from build123d import *

# Parameters (mm, degrees)
F3_W           = 1.8520833333
F3_H           = 3.7041666667
F3_H_2         = 3.175
F4_DEPTH       = 38.1
F6_DEPTH       = 25.401
F7_R           = 3.175
F8_DEPTH       = 15.24
F9_R           = 1.27
F10_DEPTH      = 22.225
F11_W          = 3.175
F11_H          = 3.81
F11_H_2        = 6.985
F12_DEPTH      = 3.175
F13_DEPTH      = 4.7625
F13_DEPTH_BACK = 3.175
F15_DEPTH      = 3.175


# Not quite as in the source:
# - a length typed as a fraction of an inch, garbled in the dataset ("3 / 203.2 mm" for 3/8 in), is restored
# - a feature names something its author has since deleted; it is built from what else it names


with BuildPart() as f1:
    # F0 (on Front) → F1 (revolve)
    with BuildSketch(Plane.XZ):
        Polygon((-38.1, 0), (-31.75, 0), (-31.75, 3.175), (-34.925, 3.175), (-34.925, 25.4), (-38.1, 25.4), align=None)
    revolve(axis=Axis((0, 0, 12.7), (0, 0, 1)))

    # F3 (on offset) → F4 (cut, symmetric)
    with BuildSketch(Plane.XZ.offset(38.1)):
        with Locations((-0.9260416667, 5.0270833333)):
            Rectangle(F3_W, F3_H)
        with Locations((0.9260416667, 5.0270833333)):
            Rectangle(F3_W, F3_H)
        with Locations((0.9260416667, 12.4354166667)):
            Rectangle(F3_W, F3_H)
        with Locations((-0.9260416667, 12.4354166667)):
            Rectangle(F3_W, F3_H)
        with Locations((-0.9260416667, 19.84375)):
            Rectangle(F3_W, F3_H)
        Polygon((1.8520833333, 3.175), (1.8520833333, 0), (50.8, 0), (50.8, 25.4), (1.8520833333, 25.4), (1.8520833333, 21.6958333333), (1.8520833333, 17.9916666667), (1.8520833333, 14.2875), (1.8520833333, 10.5833333333), (1.8520833333, 6.8791666667), align=None)
        with Locations((0.9260416667, 19.84375)):
            Rectangle(F3_W, F3_H)
        with Locations((0.9260416667, 1.5875)):
            Rectangle(F3_W, F3_H_2)
        with Locations((-0.9260416667, 1.5875)):
            Rectangle(F3_W, F3_H_2)
    extrude(amount=F4_DEPTH, both=True, mode=Mode.SUBTRACT)

    # F5 (on face) → F6 (cut, through all)
    with BuildSketch(Plane.XY.offset(25.4)):
        with BuildLine():
            ThreePointArc((0, 38.1), (3.175, 34.925), (0, 31.75))
            ThreePointArc((0, 31.75), (22.4506403027, 22.4506403027), (31.75, 0))
            Line((31.75, 0), (41.275, 0))
            ThreePointArc((41.275, 0), (27.0107441469, 31.2096992237), (-5.922835282, 40.847835282))
            Line((-5.922835282, 40.847835282), (-3.0525211735, 37.9775211735))
            ThreePointArc((-3.0525211735, 37.9775211735), (-1.5274886724, 38.0693679795), (0, 38.1))
        make_face()
    extrude(amount=-F6_DEPTH, mode=Mode.SUBTRACT)

    # F7 (on face) → F8 (join)
    with BuildSketch(Plane.XY.offset(25.4)):
        with Locations((0, 34.925)):
            Circle(F7_R)
    extrude(amount=-F8_DEPTH)

    # F9 (on face) → F10 (cut)
    with BuildSketch(Plane.XY.offset(25.4)):
        with Locations((0, 34.925)):
            Circle(F9_R)
    extrude(amount=-F10_DEPTH, mode=Mode.SUBTRACT)

    # F11 (on Right) → F12 (cut, symmetric)
    with BuildSketch(Plane.YZ):
        with Locations((36.5125, 23.495)):
            Rectangle(F11_W, F11_H)
        with Locations((33.3375, 23.495)):
            Rectangle(F11_W, F11_H)
        with Locations((36.5125, 15.875)):
            Rectangle(F11_W, F11_H)
        with Locations((36.5125, 6.6675)):
            Rectangle(F11_W, F11_H_2)
        with Locations((33.3375, 6.6675)):
            Rectangle(F11_W, F11_H_2)
        with Locations((33.3375, 15.875)):
            Rectangle(F11_W, F11_H)
    extrude(amount=F12_DEPTH, both=True, mode=Mode.SUBTRACT)

    # F3 (on offset) → F13 (join, two sides)
    with BuildSketch(Plane.XZ.offset(38.1)) as f13_sk:
        with Locations((-0.9260416667, 8.73125)):
            Rectangle(F3_W, F3_H)
        with Locations((0.9260416667, 8.73125)):
            Rectangle(F3_W, F3_H)
        with Locations((-0.9260416667, 16.1395833333)):
            Rectangle(F3_W, F3_H)
        with Locations((0.9260416667, 16.1395833333)):
            Rectangle(F3_W, F3_H)
        with Locations((-0.9260416667, 23.5479166667)):
            Rectangle(F3_W, F3_H)
        with Locations((0.9260416667, 23.5479166667)):
            Rectangle(F3_W, F3_H)
    extrude(amount=F13_DEPTH)
    extrude(f13_sk.sketch, amount=-F13_DEPTH_BACK)

    # F14 (on face) → F15 (cut)
    with BuildSketch(Plane(origin=(0, 0, 0), x_dir=(1, 0, 0), z_dir=(0, 0, -1))):
        with BuildLine():
            Line((0, -31.75), (0, -34.925))
            Line((0, -34.925), (-3.0525211735, -37.9775211735))
            ThreePointArc((-3.0525211735, -37.9775211735), (-1.5274886724, -38.0693679795), (0, -38.1))
            ThreePointArc((0, -38.1), (3.175, -34.925), (0, -31.75))
        make_face()
    extrude(amount=-F15_DEPTH, mode=Mode.SUBTRACT)


solid = f1.part
The listing builds one solid part. Answer for the finished solid, in the listing's coordinates (mm). A direction names the side the tool comes from. Round coordinates to 2 decimals unless told otherwise and drop trailing zeros. Write each loop counter-clockwise with the first axis right and the second up, starting at its lowest first coordinate (ties: lowest second). Pieces come first, ordered by that corner, then holes. Notation, with made-up numbers: M -5,72.25 L 11,72.25 A30 cw 11,108.25 Z; hole C 82,-15.75 d5. An arc over 180 degrees is marked long. Write each question's results on one line, items separated by ' | '. Start each with the question number.
Item 1: A cutting plane is placed at D-D on y = 8. Write down the section's boundary in (x, z) (3 decimals), and give its area (3 significant figures).
Item 2: Straight lines are drawn through the part: L1, parallel to Y at x = -27, z = 19.25; L2, parallel to Y at x = -6.5, z = 10.75; L3, parallel to X at y = -13, z = 8.75. For each, find the intervals that lie inside material, in ascending order. Write a range as [from, to].
Item 3: Flat-ended cylindrical pins translate along their axes: pin 1 Ø1.6 at (y, z) = (37, 23.5) entering from +X (3 decimals); pin 2 Ø12 at (x, z) = (-16.5, 12) entering from -Y; pin 3 Ø5 at (x, y) = (0, 34.5) entering from +Z; pin 4 Ø6 at (x, y) = (-19.5, 19.5) entering from -Z. Find the tip coordinate at first contact, or state that the pin passes through.
Item 4: For faces 1 (the face through (0, 33, 2)), 2 (the face through (-1.852, -40, 24)), 3 (the face through (-1.505, 36.43, 1.565)), 4 (the face through (0, 36.4, 17.78)), 5 (the face through (-1.852, -36, 20)), determine the directions among +Z, -Z, +X, -X, +Y, -Y from which every point of the face is accessible in a straight line to the end or side of a thin tool.
Item 5: A cutting plane is placed at A-A on x = -26. Write down the section's boundary in (y, z) (3 decimals).
Item 6: For a pull along Y with two mould halves and no side action, classify faces 6 (the face through (0, -42.863, 24)), 7 (the face through (-1, 36, 13.97)), 8 (the face through (2.37, 32.81, 19.71)) as pulls with the +Y half, pulls with the -Y half, needs draft (parallel to the pull), parting line crosses it, or undercut.
Item 7: A cutting plane is placed at B-B on z = 20. Write down the section's boundary in (x, y) (3 decimals), and give its area (3 significant figures).
Check sheet entries:
1) outline: M -37.251,0 L -30.726,0 L -30.726,3.175 L -33.996,3.175 L -33.996,25.4 L -37.251,25.4 Z | area: 93.0 mm²
2) L1: [-26.88, -22.15], [22.15, 26.88] | L2: [-37.54, -34.31], [34.31, 37.54] | L3: [-35.81, -32.42]
3) pin 1: x = -3.175 | pin 2: y = -36.62 | pin 3: z = 21.59 | pin 4: through
4) face 1: -Z, +X, +Y, -Y | face 2: +Z, -Z, -X, -Y | face 3: -Z, +X, +Y | face 4: +X, +Y | face 5: +X, -Y
5) outline: M -27.85,0 L -18.223,0 L -18.223,3.175 L -23.319,3.175 L -23.319,25.4 L -27.85,25.4 Z; M 18.223,0 L 27.85,0 L 27.85,25.4 L 23.319,25.4 L 23.319,3.175 L 18.223,3.175 Z
6) face 6: pulls with the -Y half | face 7: needs draft | face 8: undercut
7) outline: M -3.172,34.781 A3.175 ccw long 0,38.1 A38.1 ccw -1.852,-38.055 L -1.852,-34.876 A34.925 cw Z; hole C 0,34.925 d2.54 | area: 377 mm²
